Source: CAD feature listing. Evaluate the final solid. Frame: model axes, mm. A direction names the side the tool comes from. Give positions to 0.01 mm unless a question says otherwise; leave off trailing zeros. Order: outer loops, then holes, each group sorted by start corner. A loop starts at its lowest first (then second) coordinate and runs counter-clockwise, first axis right, second up.
1) Draft query along Y for faces 1 (the face through (6, 2.032, -17)), 2 (the face through (-12.7, 1, 0)), 3 (the face through (6, 5.182, -17)). Return one class per face: released by +Y, released by -Y, zero draft, split by the parting line, or undercut.
2) Section B-B, the plane x = 1.25. Return loops of the section in (y, z) (3 decimals), plus the area to 3 significant figures.
3) Material intervals for line 1 (Y direction, x = 6.5, z = -18); line 2 (X direction, y = 4.75, z = -19); line 3 (X direction, y = 4.75, z = -12), sorted ascending.
4) Section C-C, the plane z = -13. Give the number of separate pieces and of enclosed holes in the cut face, plus the area to 3 significant figures.
5) Access query for faces 4 (the face through (7.874, 2, 7)), 5 (the face through (9.398, 2, -17)), 6 (the face through (6, 4.928, -17)), 7 (the face through (9.97, 4, -17)), 8 (the face through (2.35, 4, -17)). Directions: +Z, -Z, +X, -X, +Y, -Y. A direction counts if a zero-diameter tool reaches every point of the face in a straight line with its end or side. Return the directions, or none.
6) Section D-D, the plane y = 6.25. Return loops of the section in (x, z) (3 decimals), plus the area to 3 significant figures.
7) Section A-A, the plane z = 10. Return loops of the section in (x, y) (3 decimals), plus the area to 3 significant figures.
8) First-contact query: P1, Ø10, axis at x = -7.5, z = 1, coming from the +Y side; P2, Ø0.5, axis at y = 2.5, z = -17, coming from the +X side; P3, Ø0.5, axis at y = 3, z = 3.5, coming from the +X side; P4, Ø1, axis at x = -1, y = 5, coming from the +Z side. Flat tips, straight axial feed; report the tip coordinate or a pass-through.
Autodesk Inventor part; units mm, degrees
ref_plane "YZ Plane" through (0, 0, 0) normal (1, 0, 0) x (0, 1, 0)
ref_plane "XZ Plane" through (0, 0, 0) normal (0, 1, 0) x (-1, 0, 0)
ref_plane "XY Plane" through (0, 0, 0) normal (0, 0, 1) x (1, 0, 0)
sketch "Sketch1" plane through (0, 0, 0) normal (0, 1, 0) x (-1, 0, 0)
  line L0 (12.7, 20.955) -> (-12.7, 20.955)
  line L1 (-12.7, 20.955) -> (-12.7, -20.955)
  line L2 (-12.7, -20.955) -> (12.7, -20.955)
  line L3 (12.7, -20.955) -> (12.7, 20.955)
  point P0 (0, 0)
  point P1 (12.7, 0)
  point P2 (0, -20.955)
  dimension "d0" = 41.91
  dimension "d1" = 25.4
extrude "Extrusion1" add sketch "Sketch1" along normal blind 1.524
sketch "Sketch2" plane through (0, 1.524, 0) normal (0, 1, 0) x (1, 0, 0)
  line L0 (-9.144, -17.653) -> (7.874, -17.653)
  line L1 (7.874, -17.653) -> (7.874, 3.937)
  line L2 (7.874, 3.937) -> (-9.144, 3.937)
  line L3 (-9.144, 3.937) -> (-9.144, -17.653)
  line L4 (12.7, -20.955) -> (12.7, 20.955)
  line L5 (-12.7, -20.955) -> (12.7, -20.955)
  point P0 (0, 0)
  dimension "d4" = 21.59
  dimension "d5" = 17.018
  dimension "d6" = 4.826
  dimension "d7" = 3.302
extrude "Extrusion2" add sketch "Sketch2" along normal blind 2.4384
fillet "Fillet1" radius 0.635 4 edges at (-0.635, 3.9624, 17.653) (7.874, 3.9624, 6.858) (-0.635, 3.9624, -3.937) (-9.144, 3.9624, 6.858)
sketch "Sketch3" plane through (0, 1.524, 0) normal (0, 1, 0) x (1, 0, 0)
  line L0 (-8.128, 11.303) -> (-2.286, 11.303)
  line L1 (-2.286, 11.303) -> (-2.286, 17.145)
  line L2 (-2.286, 17.145) -> (-8.128, 17.145)
  line L3 (-8.128, 17.145) -> (-8.128, 11.303)
  line L4 (-12.7, 20.955) -> (-12.7, -20.955)
  line L5 (12.7, 20.955) -> (-12.7, 20.955)
  point P0 (0, 0)
  dimension "d11" = 5.842
  dimension "d12" = 5.842
  dimension "d13" = 4.572
  dimension "d14" = 3.81
extrude "Extrusion3" add sketch "Sketch3" along normal blind 9.398
sketch "Sketch4" plane through (-2.286, 1.524, -17.145) normal (0, 0, -1) x (-1, 0, 0)
  circle A0 centre (2.921, 6.35) radius 2.54
  line L0 (0, 9.398) -> (5.842, 9.398)
  point P0 (-2.286, -1.524)
  point P1 (2.921, 9.398)
  dimension "d17" = 5.08
  dimension "d18" = 0.508
extrude "Extrusion4" add sketch "Sketch4" along normal blind 8.89
sketch "Sketch5" plane through (12.7, 0, -20.955) normal (0, 0, -1) x (-1, 0, 0)
  line L0 (0, 1.524) -> (25.4, 1.524)
  line L1 (3.302, 1.524) -> (9.779, 1.524)
  line L2 (9.779, 1.524) -> (9.779, 3.048)
  line L3 (3.302, 3.048) -> (3.302, 1.524)
  line L4 (2.7305, 3.048) -> (2.7305, 5.1816)
  line L5 (2.7305, 5.1816) -> (10.3505, 5.1816)
  line L6 (10.3505, 5.1816) -> (10.3505, 3.048)
  line L7 (10.3505, 3.048) -> (9.779, 3.048)
  line L8 (3.302, 3.048) -> (2.7305, 3.048)
  point P0 (12.7, 0)
  point P1 (10.0648, 3.048)
  point P2 (3.0162, 3.048)
  dimension "d21" = 3.6576
  dimension "d22" = 1.524
  dimension "d23" = 7.62
  dimension "d24" = 6.477
  dimension "d25" = 3.302
extrude "Extrusion5" add sketch "Sketch5" against normal blind 9.017
sketch "Sketch6" plane through (12.7, 0, -20.955) normal (0, 0, -1) x (-1, 0, 0)
  line L0 (0, 0) -> (25.4, 0)
  line L1 (25.4, 0) -> (25.4, 1.524)
  line L2 (9.779, 1.524) -> (25.4, 1.524)
  line L3 (9.779, 1.524) -> (9.779, 3.048)
  line L4 (9.779, 3.048) -> (10.3505, 3.048)
  line L5 (10.3505, 3.048) -> (10.3505, 5.1816)
  line L6 (10.3505, 5.1816) -> (2.7305, 5.1816)
  line L7 (2.7305, 5.1816) -> (2.7305, 3.048)
  line L8 (2.7305, 3.048) -> (3.302, 3.048)
  line L9 (3.302, 3.048) -> (3.302, 1.524)
  line L10 (0, 1.524) -> (3.302, 1.524)
  line L11 (0, 0) -> (0, 1.524)
  line L12 (2.9845, 4.9276) -> (10.0965, 4.9276)
  line L13 (10.0965, 4.9276) -> (10.0965, 3.302)
  line L14 (2.9845, 3.302) -> (2.9845, 4.9276)
  line L15 (3.302, 1.524) -> (9.779, 1.524)
  line L16 (9.525, 3.302) -> (9.525, 1.524)
  line L17 (9.525, 1.524) -> (3.556, 1.524)
  line L18 (3.556, 1.524) -> (3.556, 3.302)
  line L19 (10.0965, 3.302) -> (9.525, 3.302)
  line L20 (3.556, 3.302) -> (2.9845, 3.302)
  line L21 (4.191, 3.5052) -> (8.89, 3.5052)
  line L22 (8.89, 3.5052) -> (8.89, 2.7686)
  line L23 (8.89, 2.7686) -> (4.191, 2.7686)
  line L24 (4.191, 2.7686) -> (4.191, 3.5052)
  line L25 (4.191, 2.7686) -> (4.9276, 2.032)
  line L26 (4.191, 2.7686) -> (5.2327, 2.7686) construction
  line L27 (4.9276, 2.032) -> (8.1534, 2.032)
  line L28 (8.1534, 2.032) -> (8.89, 2.7686)
  line L29 (6.5405, 3.5052) -> (6.5405, 2.032) construction
  point P0 (12.7, 0)
  point P1 (6.5405, 2.7686)
  point P2 (6.5405, 2.7686)
  dimension "d28" = 0.254
  dimension "d29" = 0.254
  dimension "d30" = 0.254
  dimension "d32" = 0.254
  dimension "d33" = 0.254
  dimension "d34" = 0.254
  dimension "d35" = 0.254
  dimension "d36" = 45
  dimension "d37" = 0.635
  dimension "d38" = 0.635
  dimension "d39" = 0.508
  dimension "d40" = 1.4224
extrude "Extrusion6" cut sketch "Sketch6" against normal blind 8.763 contours L18 L20 L14 L12 L13 L19 L16 L15
fillet "Fillet2" radius 0.127 10 edges at (9.9695, 3.048, -16.4465) (9.398, 3.048, -16.4465) (9.7155, 3.302, -16.5735) (9.144, 3.302, -16.5735) (3.175, 3.302, -16.5735) (2.6035, 3.302, -16.5735) (2.3495, 3.048, -16.4465) (2.921, 3.048, -16.4465) (2.3495, 5.1816, -16.4465) (9.9695, 5.1816, -16.4465)
equation "\"d12\" = d11"
equation "\"d29\" = d28"
equation "\"d30\" = d28"
equation "\"d32\" = d28"
equation "\"d33\" = d28"
equation "\"d34\" = d28"
equation "\"d35\" = d28"
equation "\"d38\" = d37"
equation "\"d31\" = d28"
properties part number "GPS"
From the geometry:
1. face 1: undercut
1. face 2: zero draft
1. face 3: released by +Y
2. outline: (0, -20.955) - (1.524, -20.955) - (1.524, -3.937) - (3.327, -3.937) arc R0.635 ccw to (3.962, -3.302) - (3.962, 17.018) arc R0.635 ccw to (3.327, 17.653) - (1.524, 17.653) - (1.524, 20.955) - (0, 20.955) - close
2. area: 116 mm2
3. line 1: y = 0 to 1.52, 2.03 to 3.51, 4.93 to 5.18
3. line 2: x = 2.35 to 2.6, 9.72 to 9.97
3. line 3: x = -8.13 to -2.29, 2.35 to 9.97
4. separate pieces: 2
4. enclosed holes: 1
4. area: 104 mm2
5. face 4: +Z, +X, +Y
5. face 5: +Z, -Z, +X
5. face 6: -Z
5. face 7: +Z, -Z, +X, +Y
5. face 8: -Z, +Y
6. outline: (-8.128, -17.145) - (-7.16, -17.145) - (-7.16, -26.035) - (-3.254, -26.035) - (-3.254, -17.145) - (-2.286, -17.145) - (-2.286, -11.303) - (-8.128, -11.303) - close
6. area: 68.9 mm2
7. outline: (-12.7, 0) - (12.7, 0) - (12.7, 1.524) - (7.874, 1.524) - (7.874, 3.327) arc R0.635 ccw to (7.239, 3.962) - (-8.509, 3.962) arc R0.635 ccw to (-9.144, 3.327) - (-9.144, 1.524) - (-12.7, 1.524) - close
7. area: 80.0 mm2
8. P1: stops at y = 3.96
8. P2: stops at x = 9.4
8. P3: stops at x = 7.87
8. P4: passes through
